```python
from build123d import *

# Parameters (mm, degrees)
F0_W     = 2
F0_H     = 0.7
F1_DEPTH = 1.45
F2_SCALE = 15
F3_W     = 6
F3_H     = 11.75
F4_DEPTH = 1


with BuildPart() as f1:
    # F0 (on Front) → F1 (new body)
    with BuildSketch(Plane.XZ):
        Rectangle(F0_W, F0_H)
    extrude(amount=F1_DEPTH)


with BuildPart() as f1_1:
    # F2: moved
    add(f1.part.scale(F2_SCALE))

    # F3 (on face) → F4 (join)
    with BuildSketch(Plane.XY.offset(5.25)):
        with Locations((8, -10.875)):
            Rectangle(F3_W, F3_H)
    extrude(amount=F4_DEPTH)


solid = f1_1.part
```
Verification items for the finished model (mm, model axes). A direction names the side the tool comes from. Give positions to 0.01 mm unless a question says otherwise; leave off trailing zeros. Loops run counter-clockwise (first coordinate to the right, second up) from the corner with the lowest first, then second, coordinate; pieces in that order, holes last. Notation, with made-up numbers: M 32.5,13.5 L 73.5,13.5 A33 ccw 73.5,41.5 Z; hole C 89,73.5 d4. An arc over 180 degrees is marked long. One line per question, with ' | ' between items.
Item 1: Section check D-D, the plane y = -18.5. Record the cut outline in (x, z).
Completed:
outline: M -15,-5.25 L 15,-5.25 L 15,5.25 L -15,5.25 Z
Item 2: Section check A-A, the plane y = -13. Record the cut outline in (x, z).
Completed:
outline: M -15,-5.25 L 15,-5.25 L 15,5.25 L 11,5.25 L 11,6.25 L 5,6.25 L 5,5.25 L -15,5.25 Z
Item 3: Depth check by flat-ended pin: P1, Ø1, axis at x = -4, y = -8.5, coming from the +Z side. Enter the tip coordinate at first touch or a pass-through.
Completed:
P1: stops at z = 5.25
Item 4: Section check C-C, the plane x = -1. Record the cut outline in (y, z).
Completed:
outline: M -21.75,-5.25 L 0,-5.25 L 0,5.25 L -21.75,5.25 Z
Item 5: Tool access check on faces 1 (the face through (8, -16.75, 6)), 2 (the face through (11, -11, 6)), 3 (the face through (5, -11, 6)), 4 (the face through (8, -5, 6)). Record the directions out of +Z, -Z, +X, -X, +Y, -Y that give a thin tool (end or side, any length) a straight path to the whole face; none if there is none.
Completed:
face 1: +Z, +X, -X, -Y | face 2: +Z, +X, +Y, -Y | face 3: +Z, -X, +Y, -Y | face 4: +Z, +X, -X, +Y
Item 6: Thickness scan on line 1 (Z direction, x = -1.75, y = -6.75); line 2 (Y direction, x = 7.5, z = 5.5). Record the ranges inside material, lowest first. Write a range as [from, to].
Completed:
line 1: z = [-5.25, 5.25] | line 2: y = [-16.75, -5]
Item 7: Section check B-B, the plane x = 10. Record the cut outline in (y, z).
Completed:
outline: M -21.75,-5.25 L 0,-5.25 L 0,5.25 L -5,5.25 L -5,6.25 L -16.75,6.25 L -16.75,5.25 L -21.75,5.25 Z
